Source: CAD feature listing. Evaluate the final solid. Frame: model axes, mm. Give positions to 0.01 mm unless a question says otherwise; leave off trailing zeros. Write each loop counter-clockwise with the first axis right and the second up, starting at its lowest first coordinate (ties: lowest second). Pieces come first, ordered by that corner, then holes. Notation, with made-up numbers: M 11.25,65 L 68.25,65 A9 ccw 68.25,73 Z; hole C -29.5,11 d4. An arc over 180 degrees is marked long. Answer as a JSON object with one key per item and string values. Group by question number.
```python
from build123d import *

# Parameters (mm, degrees)
BOSS_EXTRUDE1_DEPTH = 1.5875
SKETCH2_R           = 1.5875
CUT_EXTRUDE1_DEPTH  = 2.5875


with BuildPart() as part:
    # Sketch1 → Boss-Extrude1 (new body)
    with BuildSketch(Plane(origin=(0, 0, 0), x_dir=(1, 0, 0), z_dir=(0, 1, 0))):
        Polygon((-34.11142792, 39.404580528), (-34.11142792, -10.709619472), (92.88857208, -10.709619472), (92.88857208, 68.563780528), align=None)
    extrude(amount=BOSS_EXTRUDE1_DEPTH)

    # Sketch2 → Cut-Extrude1 (cut, through all)
    with BuildSketch(Plane(origin=(0, 1.5875, 0), x_dir=(1, 0, 0), z_dir=(0, 1, 0))):
        with Locations((-18.23642792, 40.090380528)):
            Circle(SKETCH2_R)
        with Locations((-18.23642792, -7.534619472)):
            Circle(SKETCH2_R)
        with Locations((37.00857208, 47.710380528)):
            Circle(SKETCH2_R)
        with Locations((31.92857208, -3.089619472)):
            Circle(SKETCH2_R)
        with Locations((31.92857208, 24.850380528)):
            Circle(SKETCH2_R)
        with Locations((57.32857208, 40.090380528)):
            Circle(SKETCH2_R)
        with Locations((62.40857208, -7.534619472)):
            Circle(SKETCH2_R)
    extrude(amount=-CUT_EXTRUDE1_DEPTH, mode=Mode.SUBTRACT)


solid = part.part
```
(1) Section B-B, the plane y = 0.8. Return loops of the section in (x, z) (1 decimal).
(2) Section D-D, the plane x = 16. Return loops of the section in (y, z), plus the area to 3 significant figures.
(3) Pull-direction query (Z, two-part tool) for faces 1 (the cylindrical face through (36.66, 0.8, -46.16)), 2 (the flat face through (28, 1.588, -21)), 3 (the flat face through (30.28, 0.78, -54.19)); classes: pulls with the +Z half, pulls with the -Z half, needs draft (parallel to the pull), parting line crosses it, or undercut.
(4) Section C-C, the plane z = -55.5. Return loops of the section in (x, y), plus the area to 3 significant figures.
(5) Section A-A, the plane x = 57. Return loops of the section in (y, z), plus the area to 3 significant figures.
(6) Ray query, L1, parallel to Z at x = 32.5, y = 0.4; L2, parallel to X at y = 1.15, z = 3; L3, parallel to Z at x = 56, y = 0.45. Return the intervals inside material, ascending. Write a range as [from, to].
Reported:
{
 "1": {"outline": "M -34.1,-39.4 L 92.9,-68.6 L 92.9,10.7 L -34.1,10.7 Z; hole C -18.2,-40.1 d3.2; hole C -18.2,7.5 d3.2; hole C 31.9,-24.9 d3.2; hole C 31.9,3.1 d3.2; hole C 37,-47.7 d3.2; hole C 57.3,-40.1 d3.2; hole C 62.4,7.5 d3.2"},
 "2": {"outline": "M 0,-50.91 L 1.59,-50.91 L 1.59,10.71 L 0,10.71 Z", "area": "97.8 mm2"},
 "3": {"face 1": "undercut", "face 2": "needs draft", "face 3": "pulls with the -Z half"},
 "4": {"outline": "M 35.99,0 L 92.89,0 L 92.89,1.59 L 35.99,1.59 Z", "area": "90.3 mm2"},
 "5": {"outline": "M 0,-60.32 L 1.59,-60.32 L 1.59,-41.64 L 0,-41.64 Z; M 0,-38.54 L 1.59,-38.54 L 1.59,10.71 L 0,10.71 Z", "area": "108 mm2"},
 "6": {"L1": "z = [-54.7, -26.33], [-23.37, 1.61], [4.57, 10.71]", "L2": "x = [-34.11, 30.34], [33.51, 92.89]", "L3": "z = [-60.09, -40.96], [-39.22, 10.71]"}
}
